```python
from build123d import *

# Parameters (mm, degrees)
EXTRUDE_THIN1_DEPTH = 190.5
FILLET1_R           = 1.27


with BuildPart() as part:
    # Sketch1 → Extrude-Thin1 (new body)
    with BuildSketch(Plane.XY):
        with BuildLine():
            Line((6.35, 19.05), (-11.1125, 19.05))
            Line((-11.1125, 19.05), (-11.1125, 14.2875))
            ThreePointArc((-11.1125, 14.2875), (-7.672916667, 11.90625), (-6.35, 7.9375))
            Line((-6.35, 7.9375), (-6.35, 4.7625))
            Line((-6.35, 4.7625), (-4.7625, 4.7625))
            ThreePointArc((-4.7625, 4.7625), (-3.367596045, 1.394903955), (0, 0))
            Line((0, 0), (0, 1.27))
            ThreePointArc((0, 1.27), (-2.883836962, 2.792464309), (-3.253406868, 6.0325))
            Line((-3.253406868, 6.0325), (-5.08, 6.0325))
            Line((-5.08, 6.0325), (-5.08, 7.9375))
            ThreePointArc((-5.08, 7.9375), (-6.377361591, 12.27053174), (-9.8425, 15.177613949))
            Line((-9.8425, 15.177613949), (-9.8425, 17.78))
            Line((-9.8425, 17.78), (6.35, 17.78))
            Line((6.35, 17.78), (6.35, 19.05))
        make_face()
    extrude(amount=-EXTRUDE_THIN1_DEPTH)

    # Fillet1
    fillet1_edges = [part.edges().sort_by_distance(p)[0] for p in [
        (-6.35, 4.7625, -95.25),
        (-11.1125, 14.2875, -95.25),
        (-11.1125, 19.05, -95.25),
        (-3.253406868, 6.0325, -95.25),
    ]]
    fillet(fillet1_edges, radius=FILLET1_R)


solid = part.part
```
Geometry check sheet. Reference: the model listing, model coordinates, mm. A direction names the side the tool comes from. Give positions to 0.01 mm unless a question says otherwise; leave off trailing zeros. Write each loop counter-clockwise with the first axis right and the second up, starting at its lowest first coordinate (ties: lowest second). Pieces come first, ordered by that corner, then holes. Notation, with made-up numbers: (67.25, -0.5) -> (73.25, -0.5) arc R29 ccw to (73.25, 20.5) -> close; hole circle Ø8 at (82.25, 65). An arc over 180 degrees is marked (long way). One line per question, with ' | ' between items.
Item 1: Scan lines: line 1 along Y through (x, z) = (-4, -115.5); line 2 along X through (y, z) = (6.25, -138.5); line 3 along Y through (x, z) = (0.25, -36). Record each from-to range of solid material in increasing order.
Determined:
line 1: 2.18 to 5.78, 17.78 to 19.05 | line 2: -6.35 to -5.08 | line 3: 17.78 to 19.05
Item 2: Sectioned sample at B-B, the plane y = 9.5. Record the boundary of the cut face in (x, z), plus the area to 3 significant figures.
Determined:
outline: (-6.54, -190.5) -> (-5.24, -190.5) -> (-5.24, 0) -> (-6.54, 0) -> close | area: 248 mm^2
Item 3: Draft check along Y on faces 1 (the cylindrical face through (-3.4, 1.43, -93.92)), 2 (the flat face through (-2, 19.05, -94)), 3 (the cylindrical face through (-6.342, 12.217, -93.916)). Enter one of: released by +Y, released by -Y, zero draft, split by the parting line, or undercut.
Determined:
face 1: released by -Y | face 2: released by +Y | face 3: undercut
Item 4: Access from +Z, -Z, +X, -X, +Y, -Y to the whole of each face (thin tool, end or side, straight path). Record for faces 4 (the flat face through (-6.3, 11.7, 0)), 5 (the cylindrical face through (-2.442, 2.266, -93.916)).
Determined:
face 4: +Z, +X, -X, +Y, -Y | face 5: +Z, -Z, +X
Item 5: Depth check by flat-ended pin: pin 1 (1.5 mm diameter, centred on y = 7, z = -28, fed in from -X); pin 2 (0.6 mm diameter, centred on y = 0.5, z = -112.5, fed in from +X); pin 3 (3 mm diameter, centred on y = 16.5, z = -113, fed in from +X); pin 4 (6 mm diameter, centred on y = 10, z = -101, fed in from +X). Enter the tip coordinate at first touch or a pass-through.
Determined:
pin 1: x = -6.35 | pin 2: x = 0 | pin 3: x = 6.35 | pin 4: x = -5.08
